Autodesk Inventor part; units mm, degrees
ref_plane "YZ Plane" through (0, 0, 0) normal (1, 0, 0) x (0, 1, 0)
ref_plane "XZ Plane" through (0, 0, 0) normal (0, 1, 0) x (-1, 0, 0)
ref_plane "XY Plane" through (0, 0, 0) normal (0, 0, 1) x (1, 0, 0)
sketch "Sketch1" plane through (0, 0, 0) normal (1, 0, 0) x (0, 1, 0)
  line L0 (0, 0) -> (238.1897, -561.1398)
  line L1 (0, 0) -> (0, -331.1226) construction
  line L2 (0, 0) -> (11.6904, 4.9623)
  line L3 (11.6904, 4.9623) -> (249.8801, -556.1775)
  line L4 (249.8801, -556.1775) -> (238.1897, -561.1398)
  dimension "d0" = 609.6
  dimension "d2" = 23
  dimension "d3" = 12.7
extrude "Extrusion1" add sketch "Sketch1" along normal blind 304.8
sketch "Sketch2" plane through (304.8, 0, 0) normal (1, 0, 0) x (0, 0, -1)
  line L0 (0, 0) -> (561.1398, 238.1897)
  line L1 (561.1398, 0) -> (0, 238.1897)
  line L2 (561.1398, 0) -> (392.1686, 0) construction
  line L3 (4.9623, 249.8801) -> (566.102, 11.6904)
  line L4 (4.9623, 249.8801) -> (0, 238.1897)
  line L5 (561.1398, 0) -> (566.102, 11.6904)
  dimension "d6" = 23
  dimension "d7" = 12.7
  dimension "d8" = 609.6
extrude "Extrusion2" add sketch "Sketch2" along normal blind 304.8
properties part number "SeeSaw"
Work out the finished part from the listing and answer in its coordinate system (mm). A direction names the side the tool comes from. Give positions to 0.01 mm unless a question says otherwise; leave off trailing zeros. Write each loop counter-clockwise with the first axis right and the second up, starting at its lowest first coordinate (ties: lowest second). Pieces come first, ordered by that corner, then holes.
Q1. The part is cut by section A-A on z = -256. Give the vertices of the cut face in (x, y).
Answer:
outline: (0, 108.67) - (304.8, 108.67) - (304.8, 122.46) - (0, 122.46) - close; (304.8, 129.52) - (609.6, 129.52) - (609.6, 143.32) - (304.8, 143.32) - close
Q2. Given pin 1 (12 mm diameter, centred on x = 93.5, y = 149.5, fed in from -Z); pin 2 (5 mm diameter, centred on x = 168.5, z = -207.5, fed in from -Y); pin 3 (8 mm diameter, centred on x = 201, z = -174, fed in from -Y), each flat-ended and moving along its own axis, determine where each tip first touches the part or whether it passes through.
Answer:
pin 1: stops at z = -366.34
pin 2: stops at y = 87.02
pin 3: stops at y = 72.16
Q3. The part is cut by section B-B on y = 36. Give the vertices of the cut face in (x, z).
Answer:
outline: (0, -84.81) - (304.8, -84.81) - (304.8, -52.31) - (0, -52.31) - close; (304.8, -508.83) - (609.6, -508.83) - (609.6, -476.33) - (304.8, -476.33) - close
Q4. The part is cut by section C-C on x = 528. Give the vertices of the cut face in (y, z).
Answer:
outline: (0, -561.14) - (11.69, -566.1) - (249.88, -4.96) - (238.19, 0) - close
Q5. The part is cut by section D-D on x = 69.5. Give the vertices of the cut face in (y, z).
Answer:
outline: (0, 0) - (238.19, -561.14) - (249.88, -556.18) - (11.69, 4.96) - close
Q6. A tool of negligible diameter and unlimited length cuts with its end or side. For faces 1 (the face through (304.8, 63, -423)), 2 (the face through (304.8, 188, -140)), 3 (the face through (304.8, 63, -137)), 4 (the face through (609.6, 126, -282)), 5 (the face through (304.8, 188, -420)), from which of +Z, -Z, +X, -X, +Y, -Y can it reach the whole face along a straight path? Write none if from no direction.
Answer:
face 1: -Z, -X, -Y
face 2: +Z, -X, +Y
face 3: +Z, +X, -Y
face 4: +Z, -Z, +X, +Y, -Y
face 5: -Z, +X, +Y
Q7. Straight lines are drawn through the part: L1, parallel to X at y = 163, z = -195; L2, parallel to Y at x = 133, z = -433.5; L3, parallel to Z at x = 113, y = 113. For each, find the intervals that lie inside material, in ascending order.
Answer:
L1: x = 304.8 to 609.6
L2: y = 184.01 to 197.81
L3: z = -266.21 to -233.71
